from build123d import *

# Parameters (mm, degrees)
F0_W     = 71.4756
F0_H     = 37.592
F1_DEPTH = 149.86
F2_T     = -2.54
F4_D     = 6.35
F4_DEPTH = 25.4
F4_TIP   = 1.9077324654


with BuildPart() as f1:
    # F0 (on Front) → F1 (new body)
    with BuildSketch(Plane.XZ):
        with Locations((-3.4269116563, 18.796)):
            Rectangle(F0_W, F0_H)
    extrude(amount=F1_DEPTH)

    # F2
    f2_openings = [f1.faces().sort_by_distance(p)[0] for p in [
        (-3.426912, -74.93, 37.592),
    ]]
    offset(amount=F2_T, openings=f2_openings)

    # F4
    with Locations(Plane(origin=(0, 0, 0), x_dir=(1, 0, 0), z_dir=(0, 1, 0))):
        with Locations((-3.4536644816, -19.1390831023)):
            Hole(F4_D / 2, depth=F4_DEPTH)
            with Locations((0, 0, -(F4_DEPTH + F4_TIP / 2))):  # 118° drill point
                Cone(0, F4_D / 2, F4_TIP, mode=Mode.SUBTRACT)


solid = f1.part
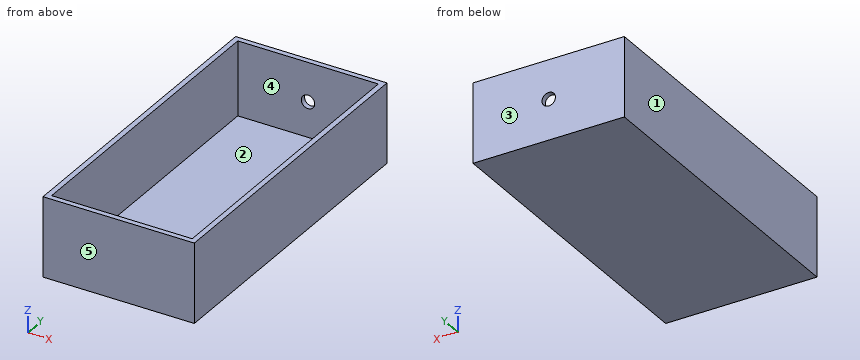
Verification items for the finished model (mm, model axes). Face numbers are marked on the shaded views. A direction names the side the tool comes from. Give positions to 0.01 mm unless a question says otherwise; leave off trailing zeros. Loops run counter-clockwise (first coordinate to the right, second up) from the corner with the lowest first, then second, coordinate; pieces in that order, holes last.
1) Draft check along X on the marked faces 1, 2 and 3. Enter one of: pulls with the +X half, pulls with the -X half, needs draft (parallel to the pull), parting line crosses it, or undercut.
2) Sectioned sample at A-A, the plane z = 32. Enter the section's corners in (x, y).
3) Sectioned sample at C-C, the plane x = -11.5. Enter the section's corners in (y, z), then the cut area to 3 significant figures.
4) Thickness scan on line 1 along Y through (x, z) = (-25, 18); line 2 along X through (y, z) = (-118, 19); line 3 along Z through (x, y) = (-8.5, -53). Record the ranges inside material, lowest first.
5) Set-up check for the marked faces 4 and 5: record each of +Z, -Z, +X, -X, +Y, -Y from which the full face is reachable in a straight line by a thin tool's end or side.
6) Depth check by flat-ended pin: pin 1 Ø5 at (x, z) = (-3.45, 19.14) entering from +Y; pin 2 Ø12 at (x, y) = (21, -61) entering from +Z. Enter the tip coordinate at first touch or a pass-through.
7) Sectioned sample at B-B, the plane y = -70. Enter the section's corners in (x, z).
Answers:
1. face 1: pulls with the -X half
1. face 2: undercut
1. face 3: needs draft
2. outline: (-39.16, -149.86) - (32.31, -149.86) - (32.31, 0) - (-39.16, 0) - close; hole (-36.62, -147.32) - (29.77, -147.32) - (29.77, -2.54) - (-36.62, -2.54) - close
3. outline: (-149.86, 0) - (0, 0) - (0, 37.59) - (-2.54, 37.59) - (-2.54, 2.54) - (-147.32, 2.54) - (-147.32, 37.59) - (-149.86, 37.59) - close
3. area: 559 mm2
4. line 1: y = -149.86 to -147.32, -2.54 to 0
4. line 2: x = -39.16 to -36.62, 29.77 to 32.31
4. line 3: z = 0 to 2.54
5. face 4: +Z
5. face 5: +Z, -Z, +X, -X, -Y
6. pin 1: stops at y = -147.32
6. pin 2: stops at z = 2.54
7. outline: (-39.16, 0) - (32.31, 0) - (32.31, 37.59) - (29.77, 37.59) - (29.77, 2.54) - (-36.62, 2.54) - (-36.62, 37.59) - (-39.16, 37.59) - close
